```python
from build123d import *

# Parameters (mm, degrees)
F1_DEPTH      = 40
F2_R          = 10
F3_DEPTH      = 180
F3_DEPTH_BACK = 20
F4_R          = 10
F5_DEPTH      = 20
F5_DEPTH_BACK = 180
F7_DEPTH      = 181.4
F9_DEPTH      = 244.2


# Not quite as in the source:
# - a feature names something its author has since deleted; it is built from what else it names


with BuildPart() as f1:
    # F0 (on Top) → F1 (new body)
    with BuildSketch(Plane.XY):
        with BuildLine():
            Line((-33.1370849898, -80), (33.1370849898, -80))
            ThreePointArc((33.1370849898, -80), (66.2741699797, -66.2741699797), (80, -33.1370849898))
            Line((80, -33.1370849898), (80, 33.1370849898))
            ThreePointArc((80, 33.1370849898), (66.2741699797, 66.2741699797), (33.1370849898, 80))
            Line((33.1370849898, 80), (-33.1370849898, 80))
            ThreePointArc((-33.1370849898, 80), (-66.2741699797, 66.2741699797), (-80, 33.1370849898))
            Line((-80, 33.1370849898), (-80, -33.1370849898))
            ThreePointArc((-80, -33.1370849898), (-66.2741699797, -66.2741699797), (-33.1370849898, -80))
        make_face()
        with BuildLine():
            Line((33.1370849898, -60), (24.8528137424, -60))
            Line((24.8528137424, -60), (-24.8528137424, -60))
            Line((-24.8528137424, -60), (-33.1370849898, -60))
            ThreePointArc((-33.1370849898, -60), (-52.132034356, -52.132034356), (-60, -33.1370849898))
            Line((-60, -33.1370849898), (-60, -24.8528137424))
            Line((-60, -24.8528137424), (-60, 24.8528137424))
            Line((-60, 24.8528137424), (-60, 33.1370849898))
            ThreePointArc((-60, 33.1370849898), (-52.132034356, 52.132034356), (-33.1370849898, 60))
            Line((-33.1370849898, 60), (-24.8528137424, 60))
            Line((-24.8528137424, 60), (24.8528137424, 60))
            Line((24.8528137424, 60), (33.1370849898, 60))
            ThreePointArc((33.1370849898, 60), (52.132034356, 52.132034356), (60, 33.1370849898))
            Line((60, 33.1370849898), (60, 24.8528137424))
            Line((60, 24.8528137424), (60, -24.8528137424))
            Line((60, -24.8528137424), (60, -33.1370849898))
            ThreePointArc((60, -33.1370849898), (52.132034356, -52.132034356), (33.1370849898, -60))
        make_face(mode=Mode.SUBTRACT)
    extrude(amount=F1_DEPTH)

    # F2 (on face) → F3 (cut, two sides)
    with BuildSketch(Plane.XZ.offset(80)) as f3_sk:
        with Locations((0, 20)):
            Circle(F2_R)
    extrude(amount=-F3_DEPTH, mode=Mode.SUBTRACT)
    extrude(f3_sk.sketch, amount=F3_DEPTH_BACK, mode=Mode.SUBTRACT)

    # F4 (on face) → F5 (cut, two sides)
    with BuildSketch(Plane.YZ.offset(80)) as f5_sk:
        with Locations((0, 20)):
            Circle(F4_R)
    extrude(amount=F5_DEPTH, mode=Mode.SUBTRACT)
    extrude(f5_sk.sketch, amount=-F5_DEPTH_BACK, mode=Mode.SUBTRACT)

    # F6 (on face) → F7 (cut)
    with BuildSketch(Plane.XZ.offset(80)):
        Polygon((-21.5, 40), (0, 40), (0, 51.6958795488), (-57.5, 51.6958795488), (-71.9271823764, 52.9654417948), (-71.9271823764, 40), (-59.4264046908, 40), (-33.1370849898, 40), align=None)
        with BuildLine():
            Line((0, 40), (0, 30))
            ThreePointArc((0, 30), (7.0710678119, 27.0710678119), (10, 20))
            Line((10, 20), (21.5, 20))
            Line((21.5, 20), (21.5, 33))
            Line((21.5, 33), (21.5, 40))
            Line((21.5, 40), (0, 40))
        make_face()
        Polygon((0, 51.6958795488), (0, 40), (21.5, 40), (21.5, 45.9314808249), (59.4264046908, 40), (71.9271823764, 40), (71.9271823764, 52.9654417948), (57.5, 51.6958795488), align=None)
        with BuildLine():
            Line((-21.5, 20), (-10, 20))
            ThreePointArc((-10, 20), (-7.0710678119, 27.0710678119), (0, 30))
            Line((0, 30), (0, 40))
            Line((0, 40), (-21.5, 40))
            Line((-21.5, 40), (-21.5, 33))
            Line((-21.5, 33), (-21.5, 20))
        make_face()
    extrude(amount=-F7_DEPTH, mode=Mode.SUBTRACT)

    # F8 (on face) → F9 (cut)
    with BuildSketch(Plane.YZ.offset(80)):
        Polygon((21.5, 0), (0, 0), (0, -11.1064584926), (57.5, -11.1064584926), (66.6687613726, -11.8878306821), (66.6687613726, 0), (59.4264046908, 0), (21.5, -5.7359817438), align=None)
        with BuildLine():
            ThreePointArc((10, 20), (7.0710678119, 12.9289321881), (0, 10))
            Line((0, 10), (0, 0))
            Line((0, 0), (21.5, 0))
            Line((21.5, 0), (21.5, 7))
            Line((21.5, 7), (21.5, 20))
            Line((21.5, 20), (10, 20))
        make_face()
        with BuildLine():
            ThreePointArc((0, 10), (-7.0710678119, 12.9289321881), (-10, 20))
            Line((-10, 20), (-21.5, 20))
            Line((-21.5, 20), (-21.5, 7))
            Line((-21.5, 7), (-21.5, 0))
            Line((-21.5, 0), (0, 0))
            Line((0, 0), (0, 10))
        make_face()
        Polygon((0, -11.1064584926), (0, 0), (-21.5, 0), (-21.5, -3.4078599419), (-59.4264046908, 0), (-66.6687613726, 0), (-66.6687613726, -11.8878306821), (-57.5, -11.1064584926), align=None)
    extrude(amount=-F9_DEPTH, mode=Mode.SUBTRACT)


solid = f1.part
```
The model under review builds one solid part; all positions refer to its coordinate system, in mm. A direction names the side the tool comes from. Coordinates: 2 decimals unless noted, no trailing zeros. Write each loop counter-clockwise with the first axis right and the second up, starting at its lowest first coordinate (ties: lowest second). Pieces come first, ordered by that corner, then holes. Notation, with made-up numbers: (47.25, -27.75) - (75.25, -27.75) arc R29 ccw to (75.25, 4.25) - close; hole circle Ø1 at (88, -23.5). An arc over 180 degrees is marked (long way). Answer in a Markdown table with one row per item. Add a question column.
Q1. Consider section C-C on y = -38. Give the boundary of the cut face in (x, z).
Q2. Draft analysis for pull direction X (two halves, no side actions). For faces 1 (the face through (-70, 21.5, 10)), 2 (the face through (-66.637, -65.908, 19.72)), 3 (the face through (-52.34, 51.92, 19.72)), state which applies: +X half, -X half, draft (parallel to the pull), parting line (faces both ways), or undercut.
Q3. To check wall thickness, follow line 1 along Y through (x, z) = (25, 24.5); line 2 along X through (y, z) = (36.5, 24.5). State the ranges of each line that lie inside material, in increasing order. Write a range as from..to.
Q4. Consider section A-A on z = 26. Give the number of separate pieces and of enclosed holes in the cut face, then the cut area to 3 significant figures.
Q5. Clearance check with flat-ended pins moving along their axes: pin 1 (9 mm diameter, centred on x = 16, y = 71, fed in from +Z); pin 2 (6 mm diameter, centred on y = 74.5, z = 30, fed in from -X); pin 3 (1 mm diameter, centred on y = 63, z = 21, fed in from +X). State where each tip first meets the part, or that it passes through.
Q6. For faces 4 (the face through (-8, -80, 11)), 5 (the face through (-1, -63, 0)), 6 (the face through (70, -21.5, 10)), 7 (the face through (-51.92, -52.34, 19.72)), 8 (the face through (21.5, -70, 30)), list the 3-axis set-ups (+Z, -Z, +X, -X, +Y, -Y) from which the entire face can be reached by the end or side of a thin tool; tool diameter is ignored.
Q7. Consider section B-B on x = -27. Give the boundary of the cut face in (y, z), then the cut area to 3 significant figures.
Q8. Consider section D-D on y = -68.5. Give the boundary of the cut face in (x, z).
Answers below:
| question | item | result |
|---|---|---|
| 1 | outline | (-79.75, 0) - (-59.56, 0) - (-59.56, 40) - (-79.75, 40) - close; (59.56, 0) - (79.75, 0) - (79.75, 40) - (59.56, 40) - close |
| 2 | face 1 | draft |
| 2 | face 2 | -X half |
| 2 | face 3 | undercut |
| 3 | line 1 | -80..-60, 60..80 |
| 3 | line 2 | -79.88..-59.79, 59.79..79.88 |
| 4 | separate pieces | 4 |
| 4 | enclosed holes | 0 |
| 4 | area | 7,570 mm² |
| 5 | pin 1 | z = 20 |
| 5 | pin 2 | x = -60.05 |
| 5 | pin 3 | x = 69.66 |
| 6 | face 4 | +Z, -Z, +X, -X, -Y |
| 6 | face 5 | -Z, +X, -X, +Y, -Y |
| 6 | face 6 | -Z, +X, -X |
| 6 | face 7 | +Z, -Z |
| 6 | face 8 | +Z, +Y, -Y |
| 7 | outline | (-80, 0) - (-60, 0) - (-60, 40) - (-80, 40) - close; (60, 0) - (80, 0) - (80, 40) - (60, 40) - close |
| 7 | area | 1,600 mm² |
| 8 | outline | (-63.89, 0) - (63.89, 0) - (63.89, 40) - (21.5, 40) - (21.5, 20) - (10, 20) arc R10 cw to (-10, 20) - (-21.5, 20) - (-21.5, 40) - (-63.89, 40) - close |
